Autodesk Fusion 360 part; units mm, degrees
sketch "Sketch1" plane through (0, 0, 0) normal (0, 0, 1) x (1, 0, 0)
  line L0 (0, -20) -> (80.18, -20)
  line L1 (80.18, -20) -> (80.18, -56.15)
  line L2 (80.18, -56.15) -> (0, -56.15)
  line L3 (0, -56.15) -> (0, -20)
  line L4 (4.39, -25.94) -> (75.79, -25.94)
  line L5 (75.79, -25.94) -> (75.79, -50.21)
  line L6 (75.79, -50.21) -> (4.39, -50.21)
  line L7 (4.39, -50.21) -> (4.39, -25.94)
  line L8 (0, -20) -> (49, -20)
  line L9 (49, -20) -> (49, -40)
  line L10 (49, -40) -> (0, -40)
  line L11 (0, -40) -> (0, -20)
  line L12 (75.79, -38.075) -> (80.18, -38.075) construction
  line L13 (40.09, -25.94) -> (40.09, -20) construction
  line L14 (7.59, -31.075) -> (72.59, -31.075)
  line L15 (72.59, -31.075) -> (72.59, -45.075)
  line L16 (72.59, -45.075) -> (7.59, -45.075)
  line L17 (7.59, -45.075) -> (7.59, -31.075)
  line L18 (7.59, -38.075) -> (4.39, -38.075) construction
  line L19 (40.09, -31.075) -> (40.09, -25.94) construction
  circle A0 centre (2.59, -22.575) radius 1.5
  line L20 (2.59, -24.075) -> (7, -24.075) construction
  line L21 (4.09, -22.575) -> (4.09, -25) construction
  circle A1 centre (77.59, -22.575) radius 1.5
  line L22 (77.59, -24.075) -> (73.18, -24.075) construction
  line L23 (76.09, -22.575) -> (76.09, -25) construction
  circle A2 centre (77.59, -53.575) radius 1.5
  line L24 (76.09, -53.575) -> (76.09, -51.15) construction
  line L25 (77.59, -52.075) -> (73.18, -52.075) construction
  line L26 (2.59, -52.075) -> (7, -52.075) construction
  line L27 (4.09, -53.575) -> (4.09, -51.15) construction
  circle A3 centre (2.59, -53.575) radius 1.5
  line L28 (4.39, -25.94) -> (4.39, -20)
  line L29 (4.39, -25.94) -> (0, -25.94)
  line L30 (4.39, -34.7) -> (0, -34.7)
  line L31 (0, -34.7) -> (0, -40)
  line L32 (0, -40) -> (4.39, -40)
  line L33 (4.39, -40) -> (4.39, -34.7)
  dimension "d1020" = 20
  dimension "d1021" = 80.18
  dimension "d1022" = 36.15
  dimension "d1023" = 24.27
  dimension "d1024" = 71.4
  dimension "d1025" = 20
  dimension "d1026" = 49
  dimension "d1027" = 65
  dimension "d1028" = 14
  dimension "d1039" = 3
  dimension "d1040" = 28
  dimension "d1041" = 72
  dimension "d1212" = 14.7
extrude "Extrude1" add sketch "Sketch1" against normal blind 1.53
extrude "Extrude2" add sketch "Sketch1" against normal blind 11 from surface at -1.53 contours L0 L4 L8 L9 L28 | L4 L7 L9 L10 L14 L17 L33 | L9 L10 L14 L17
extrude "Extrude3" add sketch "Sketch1" along normal blind 7 contours L4 L7 L9 L10 L14 L17 L33 | L4 L5 L6 L7 L9 L10 L14 L15 L16 L17 | L9 L10 L14 L15 L16 L17 | L9 L10 L14 L17
extrude "Extrude4" cut sketch "Sketch1" against normal blind 1 from surface at 7 contours L9 L10 L14 L15 L16 L17 | L9 L10 L14 L17
Check sheet for the modelled part. Datum: model origin and axes. Units: mm. A direction names the side the tool comes from. Coordinates: 2 decimals unless noted, no trailing zeros. Loops run counter-clockwise (first coordinate to the right, second up) from the corner with the lowest first, then second, coordinate; pieces in that order, holes last. Notation, with made-up numbers: (79, 39.5) -> (93, 39.5) arc R26 ccw to (93, 74.5) -> close; hole circle Ø3 at (72.25, 81.25). An arc over 180 degrees is marked (long way). Write item = value, one per line. Start each with the question number.
1. Depth check by flat-ended pin: P1, Ø10, axis at y = -43, z = -10, coming from the -X side; P2, Ø2, axis at x = 34, z = 3.5, coming from the +Y side; P3, Ø1.5, axis at y = -29.5, z = -2, coming from the -X side; P4, Ø4, axis at x = 2.59, y = -53.575, coming from the -Z side. Enter the tip coordinate at first touch or a pass-through.
2. Section check D-D on z = 5. Record the cut outline in (x, y).
3. Tool access check on faces 1 (the flat face through (75.79, -38, 3)), 2 (the flat face through (40, -38, 6)), 3 (the flat face through (4.39, -30, -7)), 4 (the flat face through (4.39, -38, 3)), 5 (the flat face through (27, -40, -7)). Record the directions out of +Z, -Z, +X, -X, +Y, -Y that give a thin tool (end or side, any length) a straight path to the whole face; none if there is none.
4. Section check B-B on y = -48. Record the cut outline in (x, z).
5. Section check C-C on x = 48. Record the cut outline in (y, z) (3 decimals).
6. Section check A-A on x = 2.59. Record the cut outline in (y, z) (3 decimals).
7. Draft check along Y on faces 6 (the flat face through (49, -30, -7)), 7 (the flat face through (41, -50.21, 3)), 8 (the cylindrical face through (2.26, -24.04, -0.75)). Enter one of: released by +Y, released by -Y, zero draft, split by the parting line, or undercut.
8. Material ranges on line 1 (Y direction, x = 77.59, z = -0.35) (3 decimals); line 2 (X direction, y = -22, z = -1); line 3 (Z direction, x = 68.5, y = -31), recorded low to high.
Responses:
q1.P1 = 4.39
q1.P2 = -25.94
q1.P3 = 0
q1.P4 = -1.53
q2.outline = (4.39, -50.21) -> (75.79, -50.21) -> (75.79, -25.94) -> (4.39, -25.94) -> close
q3.face_1 = +Z, +X, +Y, -Y
q3.face_2 = +Z
q3.face_3 = -Z, -X, +Y, -Y
q3.face_4 = +Z, -X, +Y, -Y
q3.face_5 = -Z, +X, -X, -Y
q4.outline = (0, -1.53) -> (80.18, -1.53) -> (80.18, 0) -> (75.79, 0) -> (75.79, 7) -> (4.39, 7) -> (4.39, 0) -> (0, 0) -> close
q5.outline = (-56.15, -1.53) -> (-40, -1.53) -> (-40, -12.53) -> (-20, -12.53) -> (-20, 0) -> (-25.94, 0) -> (-25.94, 7) -> (-31.075, 7) -> (-31.075, 6) -> (-45.075, 6) -> (-45.075, 7) -> (-50.21, 7) -> (-50.21, 0) -> (-56.15, 0) -> close
q6.outline = (-56.15, -1.53) -> (-55.075, -1.53) -> (-55.075, 0) -> (-56.15, 0) -> close; (-52.075, -1.53) -> (-24.075, -1.53) -> (-24.075, 0) -> (-52.075, 0) -> close; (-21.075, -1.53) -> (-20, -1.53) -> (-20, 0) -> (-21.075, 0) -> close
q7.face_6 = zero draft
q7.face_7 = released by -Y
q7.face_8 = undercut
q8.line_1 = -56.15 to -55.075, -52.075 to -24.075, -21.075 to -20
q8.line_2 = 0 to 1.2, 3.98 to 76.2, 78.98 to 80.18
q8.line_3 = -1.53 to 7
